Geometry: final body of the model. Coordinates: model frame, mm. A direction names the side the tool comes from. Give positions to 0.01 mm unless a question says otherwise; leave off trailing zeros. Loops run counter-clockwise (first coordinate to the right, second up) from the corner with the lowest first, then second, coordinate; pieces in that order, holes last. Notation, with made-up numbers: M -25,-21.5 L -21,-21.5 A21 ccw -21,-0.5 Z; hole C 55,35 d4. An arc over 180 degrees is marked long. One line per question, with ' | ' between items. Start each with the question number.
from build123d import *

# Parameters (mm, degrees)
SKETCH2_R            = 4.2
BOSS_EXTRUDE1_DEPTH  = 5
M3_CLEARANCE_HOLE1_D = 3.8


with BuildPart() as part:
    # Sketch2 → Boss-Extrude1 (new body)
    with BuildSketch(Plane.XY):
        with BuildLine():
            Line((5.061398723, -21.923326458), (37.751345105, -44.974734343))
            Line((37.751345105, -44.974734343), (55.039901019, -20.457274556))
            Line((55.039901019, -20.457274556), (22.349954637, 2.594133329))
            ThreePointArc((22.349954637, 2.594133329), (0, 12.582148727), (-22.349954637, 2.594133329))
            Line((-22.349954637, 2.594133329), (-55.039901019, -20.457274556))
            Line((-55.039901019, -20.457274556), (-37.751345105, -44.974734343))
            Line((-37.751345105, -44.974734343), (-5.061398723, -21.923326458))
            ThreePointArc((-5.061398723, -21.923326458), (0, -22.5), (5.061398723, -21.923326458))
        make_face()
        Circle(SKETCH2_R, mode=Mode.SUBTRACT)
    extrude(amount=BOSS_EXTRUDE1_DEPTH)

    # M3 Clearance Hole1 (through all)
    with Locations(Plane.XY.offset(5)):
        with Locations((-31.727258545, -10.136387926), (-20.201554602, -26.481361117), (-36.546527793, -38.00706506), (-48.072231736, -21.662091868), (31.727258545, -10.136387926), (48.072231736, -21.662091868), (20.201554544, -26.481361199), (36.546527736, -38.007065141)):
            Hole(M3_CLEARANCE_HOLE1_D / 2)


solid = part.part
Q1. Section D-D, the plane x = 41. Output: boundary loops of the cut face in (y, z).
Q2. Section B-B, the plane y = 0. Output: boundary loops of the cut face in (x, z), plus the area to 3 significant figures.
Q3. Section C-C, the plane z = 1.3. Count the separate pieces of the cut face and the enclosed holes in it, plus the area to 3 significant figures.
Q4. Set-up query: faces 1 (the cylindrical face through (46.317, -22.39, 2.465)), 2 (the flat face through (21.18, -33.29, 2.46)). Return all of +Z, -Z, +X, -X, +Y, -Y with unobstructed straight access to the full face (end or side cutting, diameter ignored); none if empty.
Q5. Section A-A, the plane x = 0. Output: boundary loops of the cut face in (y, z).
Q6. Material intervals for L1, parallel to Y at x = 0, z = 3.95; L2, parallel to X at y = -20, z = 4.85; L3, parallel to X at y = -27.5, z = 3.5, sorted ascending.
Q7. Draft query along Y for faces 3 (the cylindrical face through (-33.54, -9.57, 2.47)), 4 (the flat face through (-38.466, -8.77, 2.465)), 5 (the cylindrical face through (-36.13, -39.86, 2.47)), 6 (the flat face through (-21.635, -33.61, 2.465)). Return one class per face: released by +Y, released by -Y, zero draft, split by the parting line, or undercut.
Q8. Contact query for flat-ended pins moving along their axis: pin 1 (5 mm diameter, centred on x = 0, y = 0, fed in from -Z); pin 2 (1.5 mm diameter, centred on y = -31, z = 4, fed in from +X). Output: stop coordinate, or through.
Model answer:
1) outline: M -40.37,0 L -10.56,0 L -10.56,5 L -40.37,5 Z
2) outline: M -26.03,0 L -4.2,0 L -4.2,5 L -26.03,5 Z; M 4.2,0 L 26.03,0 L 26.03,5 L 4.2,5 Z | area: 218 mm^2
3) separate pieces: 1 | enclosed holes: 9 | area: 3,240 mm^2
4) face 1: +Z, -Z | face 2: +Z, -Z, -Y
5) outline: M -22.5,0 L -4.2,0 L -4.2,5 L -22.5,5 Z; M 4.2,0 L 12.58,0 L 12.58,5 L 4.2,5 Z
6) L1: y = -22.5 to -4.2, 4.2 to 12.58 | L2: x = -54.39 to -48.99, -47.15 to 47.15, 48.99 to 54.39 | L3: x = -50.07 to -21.81, -18.6 to -12.97, 12.97 to 18.6, 21.81 to 50.07
7) face 3: undercut | face 4: released by +Y | face 5: undercut | face 6: released by -Y
8) pin 1: passes through | pin 2: stops at x = 48.13
